For this review, use the dimensioned drawing (mm, ordinates from the lowest corner) and the shaded views. Give positions to 0.01 mm unless a question says otherwise; leave off trailing zeros. Write each loop counter-clockwise with the first axis right and the second up, starting at its lowest first coordinate (ties: lowest second). Pieces come first, ordered by that corner, then holes.
1) We need section C-C on y = 209.5. Give the boundary of the cut face in (x, z).
2) We need section B-B on z = 3.4. Give the boundary of the cut face in (x, y) (1 decimal).
3) We need section A-A on x = 45. Give the boundary of the cut face in (y, z).
4) Wall thickness on line 1 along X through (y, z) = (130, 4.9); line 2 along X through (y, z) = (116, 4.8): over which ranges is each line inside the solid? List them lowest first.
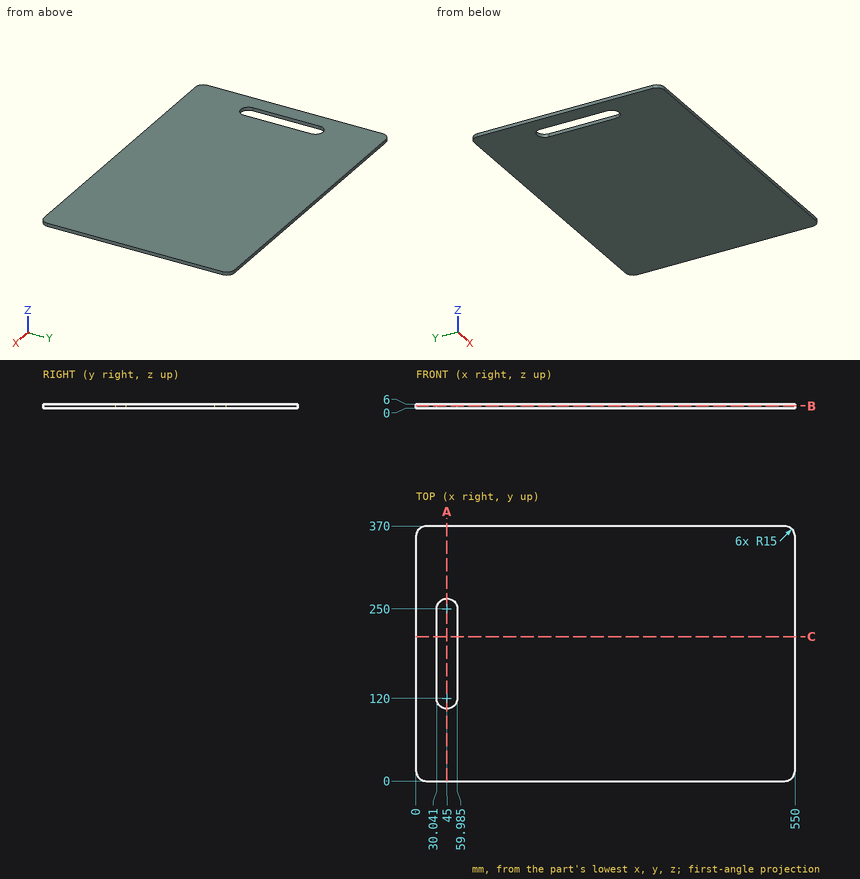
Results list:
1. outline: (0, 0) - (30.04, 0) - (30.04, 6) - (0, 6) - close; (59.99, 0) - (550, 0) - (550, 6) - (59.99, 6) - close
2. outline: (0, 15) arc R15 ccw to (15, 0) - (535, 0) arc R15 ccw to (550, 15) - (550, 355) arc R15 ccw to (535, 370) - (15, 370) arc R15 ccw to (0, 355) - close; hole (30, 118.9) arc R15 ccw to (60, 120) - (60, 249.3) arc R15 ccw to (60, 250.7) arc R15 ccw to (30, 251.1) arc R15 ccw to (30, 248.9) - (30, 121.1) arc R15 ccw to start
3. outline: (0, 0) - (105, 0) - (105, 6) - (0, 6) - close; (265, 0) - (370, 0) - (370, 6) - (265, 6) - close
4. line 1: x = 0 to 30.04, 60 to 550
4. line 2: x = 0 to 30.54, 59.46 to 550
